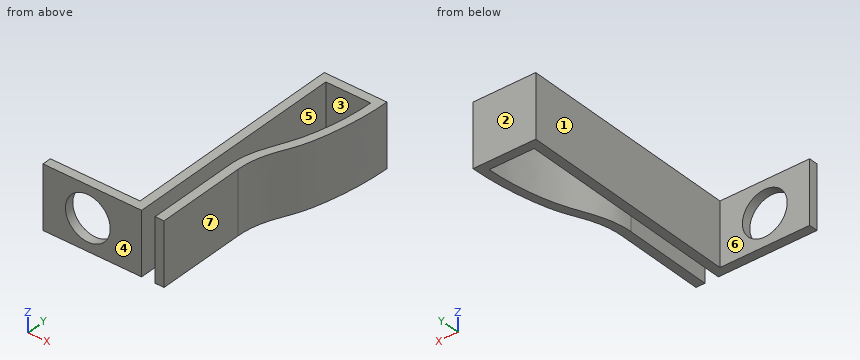
from build123d import *

# Parameters (mm, degrees)
BOSS_EXTRUDE1_DEPTH = 7
SKETCH5_R           = 2.5
CUT_EXTRUDE1_DEPTH  = 7


with BuildPart() as part:
    # Sketch1 → Boss-Extrude1 (new body)
    with BuildSketch(Plane.XY):
        with BuildLine():
            Line((0, 0), (0, 25))
            Line((0, 25), (5, 25))
            add(Edge.make_bspline(
                [(5, 25), (5, 22.505160854), (3.775153637, 15.544027487), (1.5, 13.160240213), (1.5, 10)],
                knots=[0, 0, 0, 0, 0.413095148, 1, 1, 1, 1], degree=3))
            Line((1.5, 10), (1.5, 0))
            Line((1.5, 0), (2.5, 0))
            Line((2.5, 0), (2.5, 10.023972807))
            add(Edge.make_bspline(
                [(6, 26), (6, 22.322385343), (5.041275268, 17.971400198), (3.790776866, 14.65259624), (2.5, 12.696926019), (2.5, 10.023972807)],
                knots=[0, 0, 0, 0, 0.426693592, 0.526693592, 1, 1, 1, 1], degree=3))
            Line((6, 26), (-1, 26))
            Line((-1, 26), (-1, 1))
            Line((-1, 1), (-11, 1))
            Line((-11, 1), (-11, 0))
            Line((-11, 0), (-1, 0))
            Line((-1, 0), (0, 0))
        make_face()
    extrude(amount=BOSS_EXTRUDE1_DEPTH)

    # Sketch5 → Cut-Extrude1 (cut)
    with BuildSketch(Plane(origin=(0, 1, 0), x_dir=(1, 0, 0), z_dir=(0, 1, 0))):
        with Locations(Location((-6, -3.5, 0), (0, 0, 270))):
            Circle(SKETCH5_R)
    extrude(amount=-CUT_EXTRUDE1_DEPTH, mode=Mode.SUBTRACT)


solid = part.part
Build history of the part. All positions in model axes, mm. Face numbers are marked on the shaded views. A direction names the side the tool comes from. Coordinates: 2 decimals unless noted, no trailing zeros. Write each loop counter-clockwise with the first axis right and the second up, starting at its lowest first coordinate (ties: lowest second). Pieces come first, ordered by that corner, then holes.
(1) Pin check, flat tip, straight feed: pin 1 Ø2 at (y, z) = (9.5, 4.5) entering from -X. Stop position of the tip, or through.
(2) Mould opens along Y. For the marked faces 1, 2, 3 and 4 say: pulls with the +Y half, pulls with the -Y half, needs draft (parallel to the pull), parting line crosses it, or undercut.
(3) 3-axis set-ups, long thin cutter, end or side, ignore diameter. For the marked faces 5, 6 and 7: which of +Z, -Z, +X, -X, +Y, -Y reach the whole face in a straight line?
(4) Cut at B-B on y = 4. List the corners of the cut face in (x, z).
(5) Drill centre lines: line 1 (X direction, y = 0.55, z = 3.5); line 2 (X direction, y = 9, z = 3.5); line 3 (Y direction, x = -10, z = 6.75). Where is each one in solid material? Low to high.
(6) Cut at A-A on x = -6. List the corners of the cut face in (y, z).
Working result:
1. pin 1: stops at x = -1
2. face 1: needs draft
2. face 2: pulls with the +Y half
2. face 3: undercut
2. face 4: pulls with the -Y half
3. face 5: +Z, -Z, -Y
3. face 6: +Z, -Z, -X, +Y
3. face 7: +Z, -Z, +X, -Y
4. outline: (-1, 0) - (0, 0) - (0, 7) - (-1, 7) - close; (1.5, 0) - (2.5, 0) - (2.5, 7) - (1.5, 7) - close
5. line 1: x = -11 to -8.5, -3.5 to 0, 1.5 to 2.5
5. line 2: x = -1 to 0, 1.5 to 2.5
5. line 3: y = 0 to 1
6. outline: (0, 0) - (1, 0) - (1, 1) - (0, 1) - close; (0, 6) - (1, 6) - (1, 7) - (0, 7) - close
